Part print with two shaded views. Sizes in mm from the minimum x, y, z corner. Round coordinates to 2 decimals unless told otherwise and drop trailing zeros. Loops run counter-clockwise (first coordinate to the right, second up) from the corner with the lowest first, then second, coordinate; pieces in that order, holes last.
(1) Cut at B-B on y = 6.75. List the corners of the cut face in (x, z) (1 decimal), then the cut area to 3 significant figures.
(2) Mould opens along Z. For the marked faces 1, 2, 3 and 4 say: +Z half, -Z half, draft (parallel to the pull), parting line (faces both ways), or undercut.
(3) Probe probe 1 along X at (y, z) = (13, 5.25) (1 decimal); probe 2 along Y at (x, z) = (3, 6). List the from-to ranges inside material, lowest first.
(4) Flat gauge pin, fed straight in: pin 1 (6 mm diameter, centred on y = 13, z = 8.5, fed in from -X) (3 decimals). Where does the tip first touch, or does it go through?
(5) Cut at A-A on z = 1. List the corners of the cut face in (x, y) (1 decimal), then the cut area to 3 significant figures.
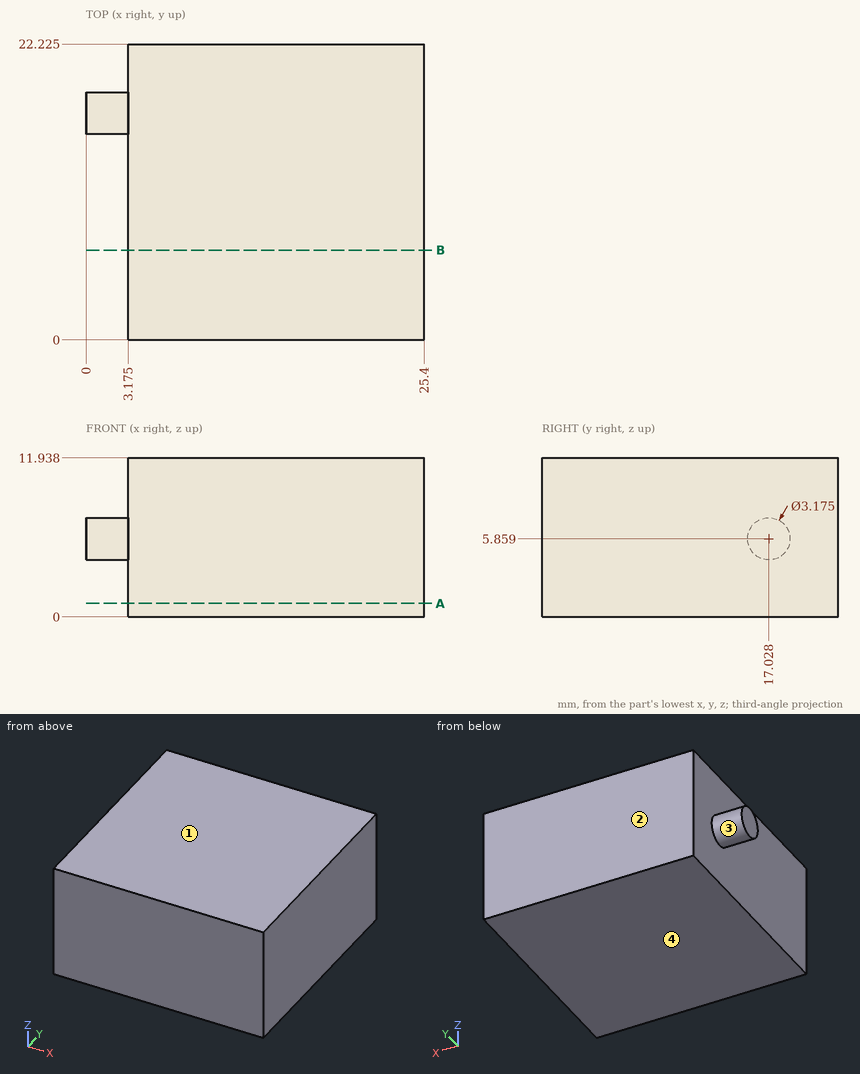
Final values:
1. outline: (3.2, 0) - (25.4, 0) - (25.4, 11.9) - (3.2, 11.9) - close
1. area: 265 mm2
2. face 1: +Z half
2. face 2: draft
2. face 3: parting line
2. face 4: -Z half
3. probe 1: x = 3.2 to 25.4
3. probe 2: y = 15.45 to 18.61
4. pin 1: stops at x = 3.175
5. outline: (3.2, 0) - (25.4, 0) - (25.4, 22.2) - (3.2, 22.2) - close
5. area: 494 mm2
